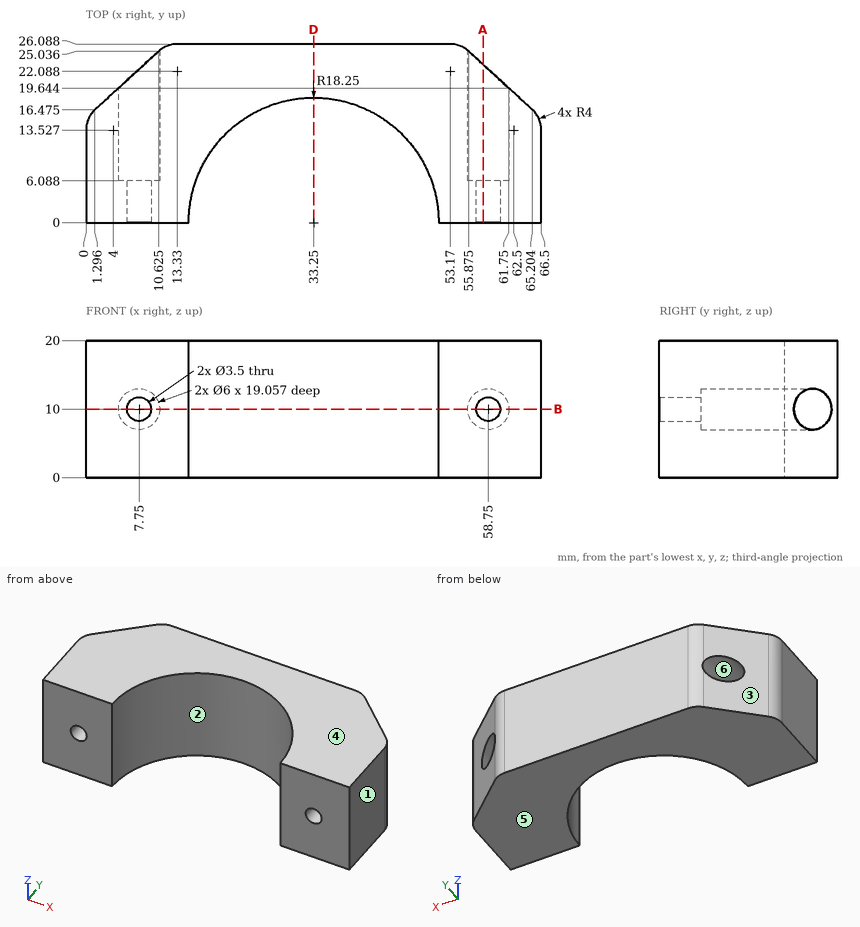
Answer from the drawing. Dimensions are ordinates in mm from the lowest x, y and z of the part. A direction names the side the tool comes from. Round coordinates to 2 decimals unless told otherwise and drop trailing zeros. Write each loop counter-clockwise with the first axis right and the second up, starting at its lowest first coordinate (ties: lowest second). Pieces come first, ordered by that corner, then holes. Notation, with made-up numbers: (8.25, -4.75) -> (50.25, -4.75) arc R11 ccw to (50.25, 9.25) -> close; hole circle Ø1 at (7.5, 86.5). An arc over 180 degrees is marked (long way). Answer in a Markdown table with one row per item. Add a question column.
1) Find section D-D, the plane x = 33.25. Determine the outline of the cut face in (y, z).
2) Find section A-A, the plane x = 58. Determine the outline of the cut face in (y, z) (1 decimal).
3) Which of the six approach directions +Z, -Z, +X, -X, +Y, -Y give full straight-line access (tool end or side, diameter ignored) to the marked faces 5 and 6?
4) Find section B-B, the plane z = 10. State how many separate pieces and enclosed holes the cut face has, and give its area (3 significant figures).
5) Given P1, Ø3, axis at x = 58.5, z = 9.5, coming from the +Y side; P2, Ø4, axis at x = 45.5, z = 14, coming from the -Y side; P3, Ø8, axis at x = 21.5, z = 10.5, coming from the -Y side, each flat-ended and moving along its own axis, determine where each tip first touches the part or whether it passes through.
6) Determine the mould class of the marked faces 1, 2, 3 and 4 for opening direction X: pulls with the +X half, pulls with the -X half, needs draft (parallel to the pull), parting line crosses it, or undercut.
7) Consider line 1 (Z direction, x = 58.75, y = 4); line 2 (X direction, y = 8.5, z = 9); line 3 (Z direction, x = 7.75, y = 15.5). Determine where each line is inside the solid, lowest interval first.
Findings below:
| question | item | result |
|---|---|---|
| 1 | outline | (18.25, 0) -> (26.09, 0) -> (26.09, 20) -> (18.25, 20) -> close |
| 2 | outline | (0, 0) -> (23.1, 0) -> (23.1, 7.1) -> (6.1, 7.1) -> (6.1, 8.4) -> (0, 8.4) -> close; (0, 11.6) -> (6.1, 11.6) -> (6.1, 12.9) -> (23.1, 12.9) -> (23.1, 20) -> (0, 20) -> close |
| 3 | face 5 | -Z, +X, -X, +Y, -Y |
| 3 | face 6 | +Y |
| 4 | separate pieces | 3 |
| 4 | enclosed holes | 0 |
| 4 | area | 845 mm² |
| 5 | P1 | y = 6.09 |
| 5 | P2 | y = 11.4 |
| 5 | P3 | y = 9.22 |
| 6 | face 1 | pulls with the +X half |
| 6 | face 2 | undercut |
| 6 | face 3 | pulls with the -X half |
| 6 | face 4 | needs draft |
| 7 | line 1 | 0 to 8.25, 11.75 to 20 |
| 7 | line 2 | 0 to 4.92, 10.58 to 17.1, 49.4 to 55.92, 61.58 to 66.5 |
| 7 | line 3 | 0 to 7, 13 to 20 |
